Check sheet for the modelled part. Datum: model origin and axes. Units: mm. A direction names the side the tool comes from. Round coordinates to 2 decimals unless told otherwise and drop trailing zeros. Loops run counter-clockwise (first coordinate to the right, second up) from the corner with the lowest first, then second, coordinate; pieces in that order, holes last. Notation, with made-up numbers: (48, 31) -> (59, 31) arc R27 ccw to (59, 48) -> close; hole circle Ø6 at (50, -18). An arc over 180 degrees is marked (long way). Use one line per item in the form item = value. Start each with the question number.
(1) Set-up check for faces 4 (the flat face through (7.737, 2.535, -2.363)), 5 (the flat face through (7.1, 2.5, -3.8)), 6 (the flat face through (-2.363, 2.535, -7.737)), 7 (the flat face through (2.363, 2.535, 7.737)): record each of +Z, -Z, +X, -X, +Y, -Y from which the full face is reachable in a straight line by a thin tool's end or side.
(2) Sectioned sample at A-A (x = 0). Record the cut outline in (y, z) (3 decimals), and give its area (3 significant figures).
(3) Sectioned sample at B-B (z = 0). Record the cut outline in (x, y) (3 decimals), and give its area (3 significant figures).
(4) Draft check along X on faces 1 (the flat face through (0.3, 5, -4.4)), 2 (the flat face through (-7.737, 2.535, 2.363)), 3 (the flat face through (-5.14, 2.54, -6.24)). Enter one of: released by +X, released by -X, zero draft, split by the parting line, or undercut.
(5) Material ranges on probe 1 along X at (y, z) = (0.6, 0) (3 decimals); probe 2 along Z at (x, y) = (6.75, 1.75); probe 3 along Z at (x, y) = (8.25, 2.05), recorded low to high. Write a range as [from, to].
from build123d import *

# Parameters (mm, degrees)
SKETCH2_R           = 6.75
BOSS_EXTRUDE1_DEPTH = 5
SKETCH3_W           = 10
SKETCH3_H           = 8
CUT_EXTRUDE1_DEPTH  = 3
FILLET1_R           = 3.5
SKETCH4_R           = 3.725
CUT_EXTRUDE2_DEPTH  = 11.006248048
BOSS_EXTRUDE2_DEPTH = 5
CIRPATTERN1_COUNT   = 16


with BuildPart() as part:
    # Sketch2 → Boss-Extrude1 (new body)
    with BuildSketch(Plane(origin=(0, 0, 0), x_dir=(1, 0, 0), z_dir=(0, 1, 0))):
        with Locations(Location((0, 0, 0), (0, 0, 270))):
            Circle(SKETCH2_R)
    extrude(amount=BOSS_EXTRUDE1_DEPTH)

    # Sketch3 → Cut-Extrude1 (cut)
    with BuildSketch(Plane(origin=(0, 5, 0), x_dir=(1, 0, 0), z_dir=(0, 1, 0))):
        Rectangle(SKETCH3_W, SKETCH3_H)
    extrude(amount=-CUT_EXTRUDE1_DEPTH, mode=Mode.SUBTRACT)

    # Fillet1
    fillet1_edges = [part.edges().sort_by_distance(p)[0] for p in [
        (5, 3.5, -4),
        (5, 3.5, 4),
        (-5, 3.5, 4),
        (-5, 3.5, -4),
    ]]
    fillet(fillet1_edges, radius=FILLET1_R)

    # Sketch4 → Cut-Extrude2 (cut, through all)
    with BuildSketch(Plane(origin=(0, 2, 0), x_dir=(1, 0, 0), z_dir=(0, 1, 0))):
        with Locations(Location((0, 0, 0), (0, 0, 270))):
            Circle(SKETCH4_R)
    extrude(amount=-CUT_EXTRUDE2_DEPTH, mode=Mode.SUBTRACT)

    # Sketch5 → Boss-Extrude2 (add)
    with BuildSketch(Plane(origin=(0, 5, 0), x_dir=(1, 0, 0), z_dir=(0, 1, 0))):
        Polygon((-1.300127145, 6.623606979), (-0.269661895, 9.441952037), (0.269661895, 9.441952037), (1.300127145, 6.623606979), align=None)
        Polygon((-0.269661895, -9.441952037), (-1.300127145, -6.623606979), (1.300127145, -6.623606979), (0.269661895, -9.441952037), align=None)
    boss_extrude2 = extrude(amount=-BOSS_EXTRUDE2_DEPTH)

    # CirPattern1: Boss-Extrude2 ×16 about axis
    cirpattern1_axis = Axis((0, 0, 0), (0, 1, 0))
    for i in range(1, CIRPATTERN1_COUNT):
        add(boss_extrude2.rotate(cirpattern1_axis, i * 360 / CIRPATTERN1_COUNT))


solid = part.part
Checks:
q1.face_4 = +X, +Y, -Y
q1.face_5 = +Y, -Y
q1.face_6 = -Z, +Y, -Y
q1.face_7 = +Z, +Y, -Y
q2.outline = (0, -9.442) -> (5, -9.442) -> (5, -4) -> (2, -4) -> (2, -3.725) -> (0, -3.725) -> close; (0, 3.725) -> (2, 3.725) -> (2, 4) -> (5, 4) -> (5, 9.442) -> (0, 9.442) -> close
q2.area = 55.5 mm2
q3.outline = (-9.442, 0) -> (-3.725, 0) -> (-3.725, 2) -> (-5, 2) -> (-5, 5) -> (-9.442, 5) -> close; (3.725, 0) -> (9.442, 0) -> (9.442, 5) -> (5, 5) -> (5, 2) -> (3.725, 2) -> close
q3.area = 49.5 mm2
q4.face_1 = zero draft
q4.face_2 = released by -X
q4.face_3 = undercut
q5.probe_1 = [-9.442, -3.725], [3.725, 9.442]
q5.probe_2 = [-6.6, -6.23], [-3.78, -1.46], [-1.25, 1.25], [1.46, 3.78], [6.23, 6.6]
q5.probe_3 = [-3.85, -2.83], [-0.71, 0.71], [2.83, 3.85]
